Source: CAD feature listing. Evaluate the final solid. Frame: model axes, mm. Face numbers are marked on the shaded views. A direction names the side the tool comes from. Give positions to 0.01 mm unless a question says otherwise; leave off trailing zeros. Order: outer loops, then holes, each group sorted by start corner. A loop starts at its lowest first (then second) coordinate and runs counter-clockwise, first axis right, second up.
```python
from build123d import *

# Parameters (mm, degrees)
SKIZZE1_W                                            = 36
SKIZZE1_H                                            = 65
AUFSATZ_LINEAR_AUSTRAGEN1_DEPTH                      = 4
SKIZZE2_W                                            = 6
SKIZZE2_H                                            = 65
SCHNITT_LINEAR_AUSTRAGEN1_DEPTH                      = 1
SKIZZE2_3_W                                          = 14
SKIZZE2_3_H                                          = 10
SCHNITT_LINEAR_AUSTRAGEN2_DEPTH                      = 5
VERRUNDUNG1_R                                        = 4
STIRNSENKUNG_F_R_M3_ZYLINDERSCHRAUBE_MIT_D           = 3.2
STIRNSENKUNG_F_R_M3_ZYLINDERSCHRAUBE_MIT_CBORE_D     = 6.5
STIRNSENKUNG_F_R_M3_ZYLINDERSCHRAUBE_MIT_CBORE_DEPTH = 2


with BuildPart() as part:
    # Skizze1 → Aufsatz-Linear austragen1 (new body)
    with BuildSketch(Plane(origin=(0, 0, 0), x_dir=(1, 0, 0), z_dir=(0, 1, 0))):
        Rectangle(SKIZZE1_W, SKIZZE1_H)
    extrude(amount=AUFSATZ_LINEAR_AUSTRAGEN1_DEPTH)

    # Skizze2 → Schnitt-Linear austragen1 (cut)
    with BuildSketch(Plane(origin=(0, 4, 0), x_dir=(1, 0, 0), z_dir=(0, 1, 0))):
        with Locations((-15, 0)):
            Rectangle(SKIZZE2_W, SKIZZE2_H)
        Polygon((18, -32.5), (18, 32.5), (12, 32.5), (12, 8.5), (4, 8.5), (4, -32.5), align=None)
    extrude(amount=-SCHNITT_LINEAR_AUSTRAGEN1_DEPTH, mode=Mode.SUBTRACT)

    # Skizze2_3 → Schnitt-Linear austragen2 (cut, through all)
    with BuildSketch(Plane(origin=(0, 4, 0), x_dir=(1, 0, 0), z_dir=(0, 1, 0))):
        Polygon((11, 32.5), (-11, 32.5), (-11, 0), (3, 0), (11, 0), align=None)
        with Locations((-4, -5)):
            Rectangle(SKIZZE2_3_W, SKIZZE2_3_H)
    extrude(amount=-SCHNITT_LINEAR_AUSTRAGEN2_DEPTH, mode=Mode.SUBTRACT)

    # Verrundung1
    verrundung1_edges = [part.edges().sort_by_distance(p)[0] for p in [
        (11, 1.5, 0),
        (-11, 2, 10),
        (3, 2, 10),
    ]]
    fillet(verrundung1_edges, radius=VERRUNDUNG1_R)

    # Stirnsenkung f_r M3 Zylinderschraube mit (through all)
    with Locations(Plane(origin=(0, 0, 0), x_dir=(-1, 0, 0), z_dir=(0, -1, 0))):
        with Locations((14.5, -28.5), (14.5, 26.5), (-14.5, 26.5), (-6.5, -28.5), (-6.5, -16.5), (-14.5, 14.5)):
            CounterBoreHole(STIRNSENKUNG_F_R_M3_ZYLINDERSCHRAUBE_MIT_D / 2, STIRNSENKUNG_F_R_M3_ZYLINDERSCHRAUBE_MIT_CBORE_D / 2, STIRNSENKUNG_F_R_M3_ZYLINDERSCHRAUBE_MIT_CBORE_DEPTH)


solid = part.part
```
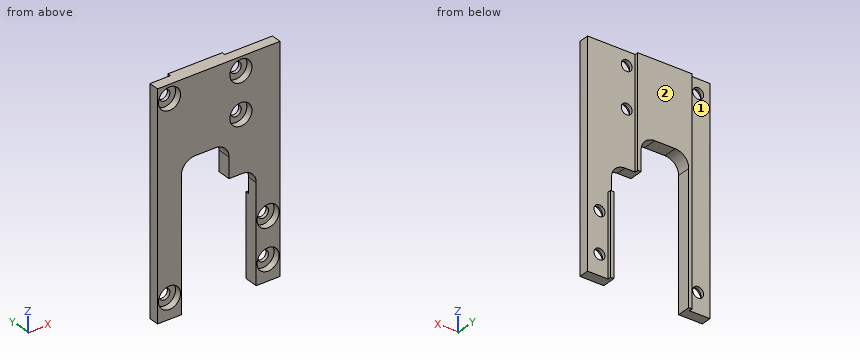
1) Section query A-A, the plane z = 16.5. Return the cut outline in (x, y), and give its area (3 significant figures).
Report:
outline: (-18, 0) - (3.25, 0) - (3.25, 2) - (4.9, 2) - (4.9, 3) - (4, 3) - (4, 4) - (-12, 4) - (-12, 3) - (-18, 3) - close; (8.1, 2) - (9.75, 2) - (9.75, 0) - (18, 0) - (18, 3) - (8.1, 3) - close
area: 108 mm2
2) Section query D-D, the plane z = 28.5. Return the cut outline in (x, y).
Report:
outline: (-18, 0) - (-17.75, 0) - (-17.75, 2) - (-16.1, 2) - (-16.1, 3) - (-18, 3) - close; (-12.9, 2) - (-11.25, 2) - (-11.25, 0) - (3.25, 0) - (3.25, 2) - (4.9, 2) - (4.9, 3) - (4, 3) - (4, 4) - (-12, 4) - (-12, 3) - (-12.9, 3) - close; (8.1, 2) - (9.75, 2) - (9.75, 0) - (18, 0) - (18, 3) - (8.1, 3) - close
3) Pin query (flat end, axial travel): pin 1 (2.5 mm diameter, centred on x = 6.5, z = 28.5, fed in from -Y); pin 2 (0.5 mm diameter, centred on y = 3.5, z = -4.5, fed in from -X); pin 3 (4 mm diameter, centred on x = 14.5, z = -26.5, fed in from +Y); pin 4 (2 mm diameter, centred on x = 15.5, z = -25.5, fed in from -Y). Return the tip coordinate at first contact, or that it passes through.
Report:
pin 1: passes through
pin 2: stops at x = -12
pin 3: stops at y = 3
pin 4: stops at y = 2
4) Section query B-B, the plane x = 14.5. Return the cut outline in (y, z).
Report:
outline: (0, -32.5) - (3, -32.5) - (3, -28.1) - (2, -28.1) - (2, -29.75) - (0, -29.75) - close; (0, -23.25) - (2, -23.25) - (2, -24.9) - (3, -24.9) - (3, -16.1) - (2, -16.1) - (2, -17.75) - (0, -17.75) - close; (0, -11.25) - (2, -11.25) - (2, -12.9) - (3, -12.9) - (3, 32.5) - (0, 32.5) - close
5) Reachability of the marked faces 1 and 2 from +Z, -Z, +X, -X, +Y, -Y: full face, straight path, thin tool, end or side. Return the list, or none.
Report:
face 1: +Z, -Z, -X, +Y
face 2: +Z, -Z, +X, -X, +Y
6) Material intervals for L1, parallel to Z at x = 14.5, y = 2.75; L2, parallel to X at y = 0.8, z = 28.5; L3, parallel to X at y = 2.85, z = -26.5, sorted ascending.
Report:
L1: z = -32.5 to -28.1, -24.9 to -16.1, -12.9 to 32.5
L2: x = -18 to -17.75, -11.25 to 3.25, 9.75 to 18
L3: x = -18 to -16.1, -12.9 to -11, 11 to 12.9, 16.1 to 18
7) Section query C-C, the plane z = -14.5. Return the cut outline in (x, y).
Report:
outline: (-18, 0) - (-11, 0) - (-11, 4) - (-12, 4) - (-12, 3) - (-18, 3) - close; (11, 0) - (11.25, 0) - (11.25, 2) - (12.9, 2) - (12.9, 3) - (12, 3) - (12, 4) - (11, 4) - close; (16.1, 2) - (17.75, 2) - (17.75, 0) - (18, 0) - (18, 3) - (16.1, 3) - close
